Check sheet for the drawn part. Datum: minimum x, y, z corner. Units: mm. Give positions to 0.01 mm unless a question says otherwise; leave off trailing zeros. Write each loop counter-clockwise with the first axis right and the second up, starting at its lowest first coordinate (ties: lowest second). Pieces come first, ordered by that corner, then holes. Notation, with made-up numbers: M 34,25.5 L 53,25.5 A27 cw 53,52.5 Z; hole C 52.5,25 d9. An arc over 180 degrees is marked long. Use CSV: the item, a comma, the result in double quotes. Start each with the question number.
1. Cross-section at C-C, the plane y = 28. Enter the section's corners in (x, z), and give its area (3 significant figures).
2. Depth check by flat-ended pin: P1, Ø1.6, axis at y = 30, z = 8.5, coming from the -X side; P2, Ø0.8, axis at x = 0.5, z = 9.5, coming from the +Y side; P3, Ø1.6, axis at x = 81, z = 6, coming from the -Y side. Enter the tip coordinate at first touch or a pass-through.
3. Scan lines: line 1 (Y direction, x = 42, z = 13.5); line 2 (X direction, y = 6, z = 13); line 3 (Y direction, x = 53, z = 0.5). Record each from-to range of solid material in increasing order.
4. Mould release check, pull along Y, two halves, no side actions. Record for the marked faces 1, 2, 3 and 4: +Y half, -Y half, draft (parallel to the pull), parting line (faces both ways), or undercut.
5. Cross-section at A-A, the plane z = 15.25. Enter the section's corners in (x, y), and give its area (3 significant figures).
6. Cross-section at B-B, the plane x = 69. Enter the section's corners in (y, z), and give its area (3 significant figures).
7. Cross-section at D-D, the plane x = 38. Enter the section's corners in (y, z), and give its area (3 significant figures).
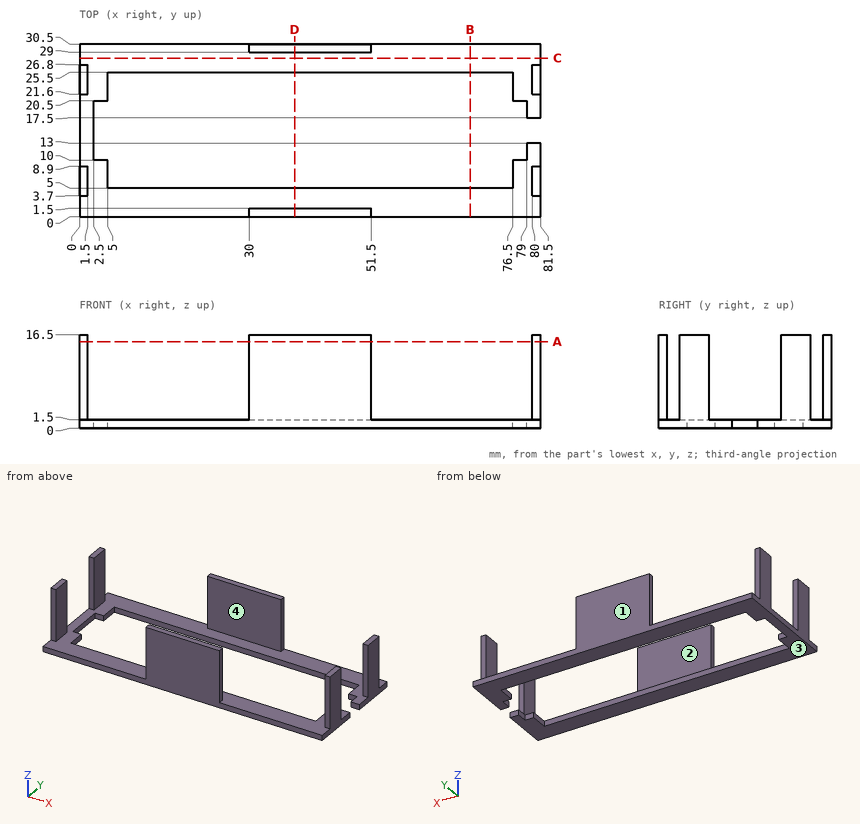
Worked answers:
1,outline,"M 0,0 L 81.5,0 L 81.5,1.5 L 0,1.5 Z"
1,area,"122 mm^2"
2,P1,"stops at x = 30"
2,P2,"stops at y = 26.8"
2,P3,"stops at y = 3.7"
3,line 1,"y = 0 to 1.5, 29 to 30.5"
3,line 2,"x = 0 to 1.5, 80 to 81.5"
3,line 3,"y = 0 to 5, 25.5 to 30.5"
4,face 1,"+Y half"
4,face 2,"undercut"
4,face 3,"draft"
4,face 4,"undercut"
5,outline,"M 0,3.7 L 1.5,3.7 L 1.5,8.9 L 0,8.9 Z; M 0,21.6 L 1.5,21.6 L 1.5,26.8 L 0,26.8 Z; M 30,0 L 51.5,0 L 51.5,1.5 L 30,1.5 Z; M 30,29 L 51.5,29 L 51.5,30.5 L 30,30.5 Z; M 80,3.7 L 81.5,3.7 L 81.5,8.9 L 80,8.9 Z; M 80,21.6 L 81.5,21.6 L 81.5,26.8 L 80,26.8 Z"
5,area,"95.7 mm^2"
6,outline,"M 0,0 L 5,0 L 5,1.5 L 0,1.5 Z; M 25.5,0 L 30.5,0 L 30.5,1.5 L 25.5,1.5 Z"
6,area,"15.0 mm^2"
7,outline,"M 0,0 L 5,0 L 5,1.5 L 1.5,1.5 L 1.5,16.5 L 0,16.5 Z; M 25.5,0 L 30.5,0 L 30.5,16.5 L 29,16.5 L 29,1.5 L 25.5,1.5 Z"
7,area,"60.0 mm^2"
